from build123d import *

# Parameters (mm, degrees)
SKETCH1_W           = 2.9
SKETCH1_H           = 15
BOSS_EXTRUDE1_DEPTH = 80
SKETCH2_W           = 6
SKETCH2_H           = 55
CUT_EXTRUDE1_DEPTH  = 80
CUT_EXTRUDE4_DEPTH  = 55


# Read off the part's stored shape, not the designer's step: Loft2
with BuildPart() as part:
    # Sketch1 → Boss-Extrude1 (new body)
    with BuildSketch(Plane(origin=(0, 0, 0), x_dir=(1, 0, 0), z_dir=(0, 1, 0))):
        Rectangle(SKETCH1_W, SKETCH1_H)
    extrude(amount=BOSS_EXTRUDE1_DEPTH)

    # Sketch2 → Cut-Extrude1 (cut)
    with BuildSketch(Plane(origin=(1.45, 0, 0), x_dir=(0, 0, -1), z_dir=(1, 0, 0))):
        with Locations((-4.5, 52.5)):
            Rectangle(SKETCH2_W, SKETCH2_H)
        with Locations((4.5, 52.5)):
            Rectangle(SKETCH2_W, SKETCH2_H)
    extrude(amount=-CUT_EXTRUDE1_DEPTH, mode=Mode.SUBTRACT)

    # Sketch3 → Cut-Extrude4 (cut)
    with BuildSketch(Plane(origin=(0, 80, 0), x_dir=(1, 0, 0), z_dir=(0, 1, 0))):
        with BuildLine():
            Line((-1.45, 1.5), (-1.45, 5e-09))
            ThreePointArc((-1.45, 5e-09), (3e-09, 1.45), (1.45, 0))
            Line((1.45, 0), (1.45, 1.5))
            Line((1.45, 1.5), (-1.45, 1.5))
        make_face()
        with BuildLine():
            Line((-1.45, 5e-09), (-1.45, -1.5))
            Line((-1.45, -1.5), (1.45, -1.5))
            Line((1.45, -1.5), (1.45, 0))
            ThreePointArc((1.45, 0), (-3e-09, -1.45), (-1.45, 5e-09))
        make_face()
    extrude(amount=-CUT_EXTRUDE4_DEPTH, mode=Mode.SUBTRACT)

    # Loft2 outline → Loft2 (revolve)
    with BuildSketch(Plane.XY):
        Polygon((1.45, 80), (0, 95), (0, 80), align=None)
    revolve(axis=Axis((0, 0, 0), (0, 1, 0)))


solid = part.part
Source: CAD feature listing. Evaluate the final solid. Frame: model axes, mm. A direction names the side the tool comes from. Give positions to 0.01 mm unless a question says otherwise; leave off trailing zeros. Order: outer loops, then holes, each group sorted by start corner. A loop starts at its lowest first (then second) coordinate and runs counter-clockwise, first axis right, second up. Notation, with made-up numbers: (-31.5, 15.5) -> (18.5, 15.5) arc R13 ccw to (18.5, 37.5) -> close; hole circle Ø7 at (79, 16). An arc over 180 degrees is marked (long way). Use a Markdown table: item, result.
1) Ray query, line 1 along Z through (x, y) = (0.15, 46.5); line 2 along Y through (x, z) = (1.3, -3.5); line 3 along Z through (x, y) = (0.85, 75). Return the intervals inside material, ascending. Write a range as [from, to].
Answer list:
| item | result |
|---|---|
| line 1 | [-1.44, 1.44] |
| line 2 | [0, 25] |
| line 3 | [-1.17, 1.17] |
2) Reachability of faces 1 (the flat face through (0, 12, 7.5)), 2 (the cylindrical face through (-1.38, 52.89, -0.44)) from +Z, -Z, +X, -X, +Y, -Y: full face, straight path, thin tool, end or side. Return the list, or none.
Answer list:
| item | result |
|---|---|
| face 1 | +Z, +X, -X, +Y, -Y |
| face 2 | +Y |
3) Section query A-A, the plane y = 68. Return the cut outline in (x, z), then the cut area to 3 significant figures.
Answer list:
| item | result |
|---|---|
| outline | circle Ø2.9 at (0, 0) |
| area | 6.61 mm² |
4) Section query B-B, the plane z = -2.25. Return the cut outline in (x, y), then the cut area to 3 significant figures.
Answer list:
| item | result |
|---|---|
| outline | (-1.45, 0) -> (1.45, 0) -> (1.45, 25) -> (-1.45, 25) -> close |
| area | 72.5 mm² |
5) Contact query for flat-ended pins moving along their axis: P1, Ø1.5, axis at x = 0, z = -4.5, coming from the +Y side; P2, Ø1, axis at x = -0.5, y = 35, coming from the +Z side. Output: stop coordinate, or through.
Answer list:
| item | result |
|---|---|
| P1 | y = 25 |
| P2 | z = 1.45 |
